Study the drawing (mm; zero at the part's minimum x, y, z) and answer. A direction names the side the tool comes from. Coordinates: 2 decimals unless noted, no trailing zeros. Loops run counter-clockwise (first coordinate to the right, second up) from the corner with the lowest first, then second, coordinate; pieces in that order, holes last. Notation, with made-up numbers: (14.25, 28.25) -> (23.25, 28.25) arc R16 cw to (23.25, 44.25) -> close; hole circle Ø9 at (82, -25). An arc over 180 degrees is marked (long way). Answer as a JSON object with one key per item and string values. Group by question number.
Q1. Each of these flat-tipped pins is pushed along its axis until it touches: P1, Ø3, axis at x = 5, y = 6, coming from the +Z side; P2, Ø2, axis at x = 29, y = 3, coming from the +Z side (1 decimal); P3, Ø5.5, axis at x = 6.5, y = 7, coming from the +Z side (1 decimal); P4, Ø2, axis at y = 9.5, z = 10, coming from the -X side. Where does it stop, or does it pass through?
Q2. The part is cut by section A-A on z = 24.63. Write down the section's boundary in (x, y) (1 decimal).
Q3. For the marked faces 5, 6 and 7, determine the directions among +Z, -Z, +X, -X, +Y, -Y from which every point of the face is accessible in a straight line to the end or side of a thin tool.
Q4. Straight lines are drawn through the part: line 1 along Y through (x, z) = (5.5, 2) (1 decimal); line 2 along Z through (x, y) = (2, 10.75); line 3 along X through (y, z) = (8.25, 20.5) (1 decimal). For each, find the intervals that lie inside material, in ascending order. Write a range as [from, to].
Q5. The part is cut by section B-B on x = 5. Write down the section's boundary in (y, z).
Q6. The part is cut by section C-C on y = 6. State how many separate pieces and enclosed holes the cut face has.
Q7. Determine the mould class of the marked faces 1, 2, 3 and 4 for opening direction X: released by +X, released by -X, zero draft, split by the parting line, or undercut.
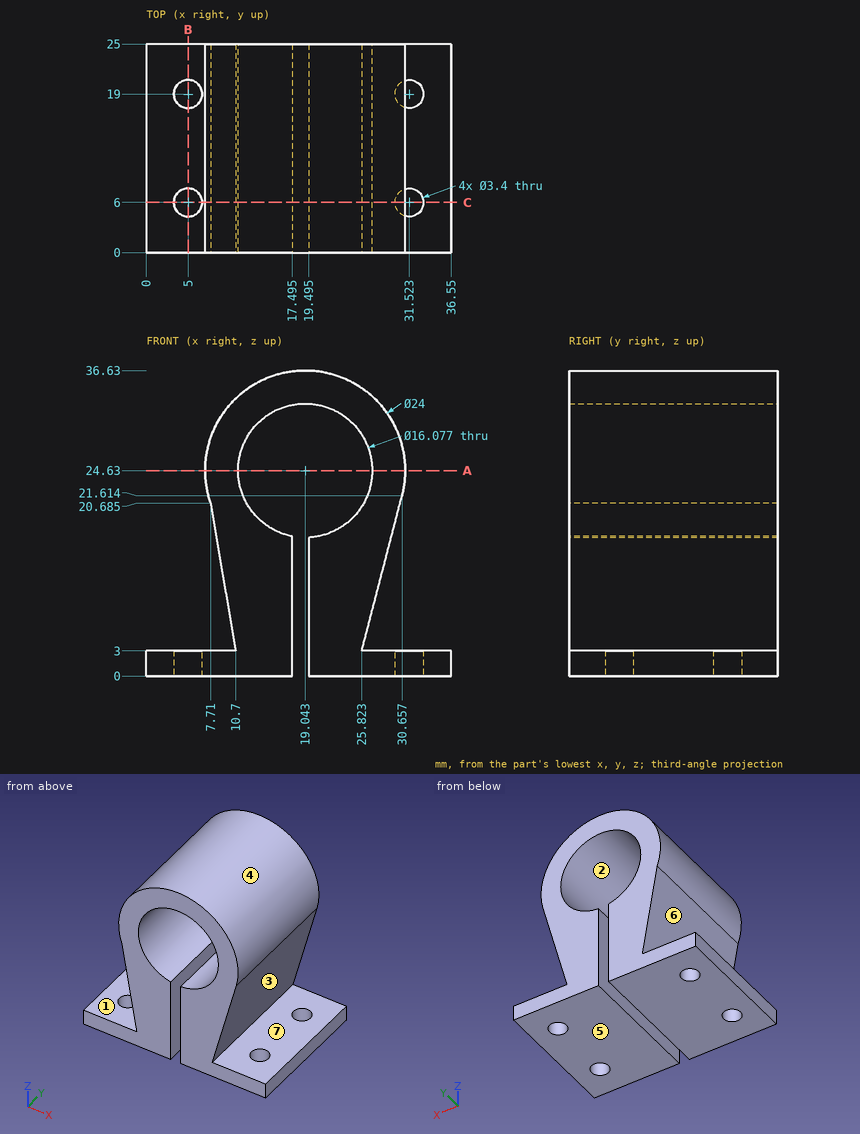
Final values:
{
 "1": {"P1": "passes through", "P2": "stops at z = 32.6", "P3": "stops at z = 31.6", "P4": "stops at x = 9.35"},
 "2": {"outline": "(7, 0) -> (11, 0) -> (11, 25) -> (7, 25) -> close; (27.1, 0) -> (31, 0) -> (31, 25) -> (27.1, 25) -> close"},
 "3": {"face 5": "-Z, +X, -X, +Y, -Y", "face 6": "-X, +Y, -Y", "face 7": "+X, +Y, -Y"},
 "4": {"line 1": "y = [0, 4.4], [7.6, 17.4], [20.6, 25]", "line 2": "z = [0, 3]", "line 3": "x = [7.7, 12.1], [25.9, 30.4]"},
 "5": {"outline": "(0, 0) -> (4.3, 0) -> (4.3, 3) -> (0, 3) -> close; (7.7, 0) -> (17.3, 0) -> (17.3, 3) -> (7.7, 3) -> close; (20.7, 0) -> (25, 0) -> (25, 3) -> (20.7, 3) -> close"},
 "6": {"separate pieces": "3", "enclosed holes": "0"},
 "7": {"face 1": "zero draft", "face 2": "undercut", "face 3": "released by +X", "face 4": "split by the parting line"}
}
